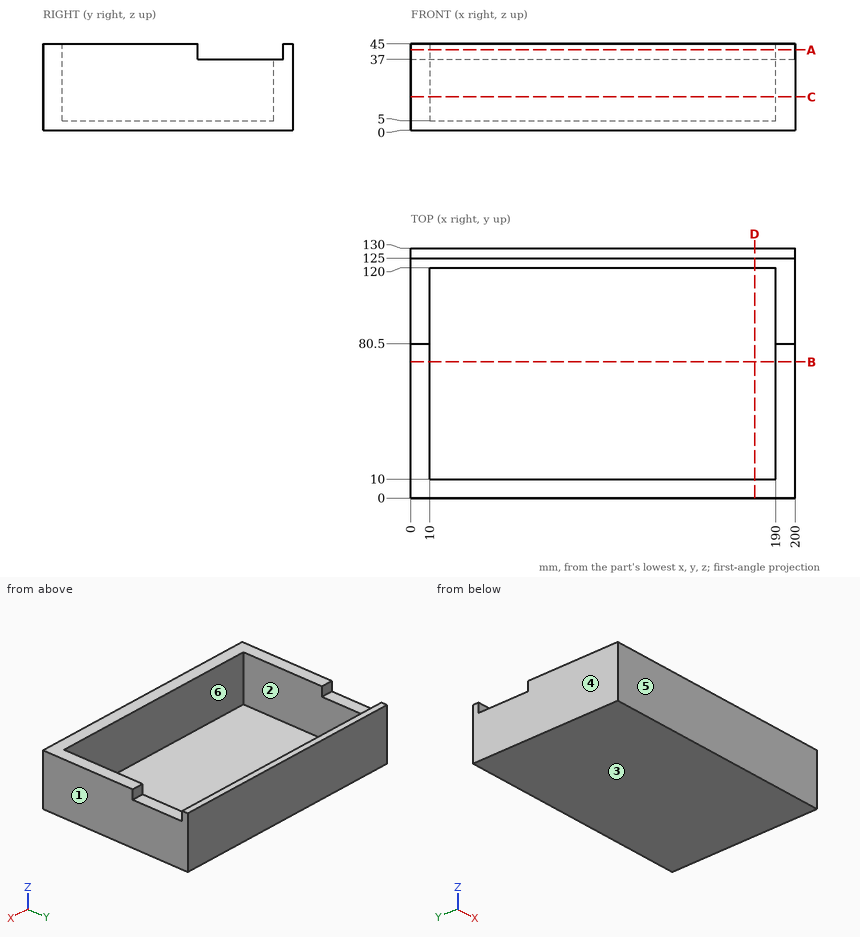
Here's the drawing with two shaded views (mm, measured from the low corner). I have some questions. A direction names the side the tool comes from. Give positions to 0.01 mm unless a question says otherwise; leave off trailing zeros. Loops run counter-clockwise (first coordinate to the right, second up) from the corner with the lowest first, then second, coordinate; pieces in that order, holes last. Notation, with made-up numbers: (52.5, 57) - (84.5, 57) arc R18 cw to (84.5, 66) - close; hole circle Ø1 at (-7.75, 16). An arc over 180 degrees is marked (long way). Answer in a Markdown table with one row per item. Add a question column.
Q1. If we section it at B-B (y = 71): List the corners of the cut face in (x, z) for me, plus the area to 3 significant figures.
Q2. Which directions (+Z, -Z, +X, -X, +Y, -Y) give clear straight access to the entire face, cutting with the end or side of a thin tool? Please do the marked faces 5 and 6.
Q3. Please list where these lines run through material, in increasing order: L1, parallel to Y at x = 31, z = 12.5; L2, parallel to X at y = 44, z = 16.5; L3, parallel to Y at x = 123.5, z = 38. Write a range as from..to.
Q4. For pin 1 (12 mm diameter, centred on x = 26.5, y = 45, fed in from +Z), with a flat end and sliding along its axis, tell me the tip position at first contact or that it passes through.
Q5. If we section it at A-A (z = 42): List the corners of the cut face in (x, y) for me.
Q6. If we section it at C-C (z = 17.5): List the corners of the cut face in (x, y) for me.
Q7. If we section it at D-D (x = 179): List the corners of the cut face in (y, z) for me.
Q8. We'd pull the mould along X, two halves only. Please class the marked faces 1, 2, 3 and 4: +X half, -X half, draft (parallel to the pull), parting line (faces both ways), or undercut.
The answers:
| question | item | result |
|---|---|---|
| 1 | outline | (0, 0) - (200, 0) - (200, 45) - (190, 45) - (190, 5) - (10, 5) - (10, 45) - (0, 45) - close |
| 1 | area | 1,800 mm^2 |
| 2 | face 5 | +Z, -Z, +X, -X, -Y |
| 2 | face 6 | +Z |
| 3 | L1 | y = 0..10, 120..130 |
| 3 | L2 | x = 0..10, 190..200 |
| 3 | L3 | y = 0..10, 125..130 |
| 4 | pin 1 | stops at z = 5 |
| 5 | outline | (0, 0) - (200, 0) - (200, 80.5) - (190, 80.5) - (190, 10) - (10, 10) - (10, 80.5) - (0, 80.5) - close; (0, 125) - (200, 125) - (200, 130) - (0, 130) - close |
| 6 | outline | (0, 0) - (200, 0) - (200, 130) - (0, 130) - close; hole (10, 10) - (190, 10) - (190, 120) - (10, 120) - close |
| 7 | outline | (0, 0) - (130, 0) - (130, 45) - (125, 45) - (125, 37) - (120, 37) - (120, 5) - (10, 5) - (10, 45) - (0, 45) - close |
| 8 | face 1 | +X half |
| 8 | face 2 | undercut |
| 8 | face 3 | draft |
| 8 | face 4 | -X half |
